Source: CAD feature listing. Evaluate the final solid. Frame: model axes, mm. A direction names the side the tool comes from. Give positions to 0.01 mm unless a question says otherwise; leave off trailing zeros. Write each loop counter-clockwise with the first axis right and the second up, starting at its lowest first coordinate (ties: lowest second). Pieces come first, ordered by that corner, then holes. Notation, with made-up numbers: M 5.5,15.25 L 28.5,15.25 A14 ccw 28.5,20.25 Z; hole C -31.75,9 d11. An arc over 180 degrees is marked long. Return JSON: item names as keys, results as strings.
Solid Edge part; units mm, degrees
sketch "Sketch1" plane through (0, 0, 0) normal (0, 0, 1) x (1, 0, 0)
  line L0 (-9, -4) -> (9, -4)
  line L1 (9, 4) -> (-9, 4)
  arc A0 (-9, 4) -> (-9, -4) centre (-9, 0) ccw
  arc A1 (9, -4) -> (9, 4) centre (9, 0) ccw
extrude "Protrusion1" add sketch "Sketch1" along normal blind 2
sketch "Sketch2" plane through (0, 0, 2) normal (0, 0, 1) x (1, 0, 0)
  circle A0 centre (9, 0) radius 1.5
extrude "Cutout1" cut sketch "Sketch2" against normal up to next
sketch "Sketch3" plane through (0, 0, 2) normal (0, 0, 1) x (1, 0, 0)
  circle A0 centre (-9, 0) radius 4
extrude "body_head_screw" add sketch "Sketch3" along normal blind 2
sketch "Sketch4" plane through (-9, 0, 4) normal (0, 0, 1) x (1, 0, 0)
  circle A0 centre (0, 0) radius 1.5
extrude "Cutout2" cut sketch "Sketch4" against normal up to next
sketch "Sketch5" plane through (-9, 0, 4) normal (0, 0, 1) x (1, 0, 0)
  line L0 (-3, 0) -> (-1.5, 2.5981)
  line L1 (-1.5, 2.5981) -> (1.5, 2.5981)
  line L2 (1.5, 2.5981) -> (3, 0)
  line L3 (3, 0) -> (1.5816, -2.5492)
  line L4 (1.5816, -2.5492) -> (-1.5816, -2.5492)
  line L5 (-3, 0) -> (-1.5816, -2.5492)
extrude "fix_screw_head" cut sketch "Sketch5" against normal blind 2
1) Draft query along X for faces 1 (the face through (7.8, -0.9, 1)), 2 (the face through (13, 0, 1)), 3 (the face through (0, -4, 1)). Return one class per face: released by +X, released by -X, zero draft, split by the parting line, or undercut.
Numbers:
{"face 1": "undercut", "face 2": "released by +X", "face 3": "zero draft"}
2) Cut plane D-D, the plane x = 5.5. Return the cut outline in (y, z).
Numbers:
{"outline": "M -4,0 L 4,0 L 4,2 L -4,2 Z"}
3) Line query: line 1 (Y direction, x = -9, z = 1.3); line 2 (Z direction, x = 8.5, y = 2.5); line 3 (Y direction, x = 8.25, z = 1.65). Output: solid intervals per line, ascending. Write a range as [from, to].
Numbers:
{"line 1": "y = [-4, -1.5], [1.5, 4]", "line 2": "z = [0, 2]", "line 3": "y = [-4, -1.3], [1.3, 4]"}
4) Cut plane A-A, the plane y = -1. Return the cut outline in (x, z), then the cut area to 3 significant figures.
Numbers:
{"outline": "M -12.87,0 L -10.12,0 L -10.12,2 L -11.44,2 L -11.44,4 L -12.87,4 Z; M -7.88,0 L 7.88,0 L 7.88,2 L -5.13,2 L -5.13,4 L -6.56,4 L -6.56,2 L -7.88,2 Z; M 10.12,0 L 12.87,0 L 12.87,2 L 10.12,2 Z", "area": "48.3 mm²"}
5) Contact query for flat-ended pins moving along their axis: pin 1 Ø1.5 at (y, z) = (2, 2.5) entering from -X; pin 2 Ø3.5 at (x, y) = (-9, 0) entering from +Z; pin 3 Ø2 at (y, z) = (1, 3.5) entering from +X. Output: stop coordinate, or through.
Numbers:
{"pin 1": "stops at x = -12.8", "pin 2": "stops at z = 2", "pin 3": "stops at x = -5"}
6) Set-up query: faces 4 (the face through (-10.5, 0.07, 1.01)), 5 (the face through (-9, -2.549, 3)). Return all of +Z, -Z, +X, -X, +Y, -Y with unobstructed straight access to the full face (end or side cutting, diameter ignored); none if empty.
Numbers:
{"face 4": "+Z, -Z", "face 5": "+Z"}
7) Cut plane B-B, the plane z = 2.6. Return the cut outline in (x, y).
Numbers:
{"outline": "C -9,0 d8; hole M -12,0 L -10.58,-2.55 L -7.42,-2.55 L -6,0 L -7.5,2.6 L -10.5,2.6 Z"}
8) Cut plane C-C, the plane z = 0.8. Return the cut outline in (x, y).
Numbers:
{"outline": "M -9,-4 L 9,-4 A4 ccw 9,4 L -9,4 A4 ccw Z; hole C -9,0 d3; hole C 9,0 d3"}
